from build123d import *

# Parameters (mm, degrees)
SKETCH1_R             = 5.5
SKETCH1_R_2           = 4.5
BOSS_EXTRUDE1_DEPTH   = 14
SKETCH1_R_3           = 3.5
SKETCH1_R_4           = 2.5
BOSS_EXTRUDE1_2_DEPTH = 14
SKETCH1_3_W           = 12
SKETCH1_3_H           = 11.5
BOSS_EXTRUDE2_DEPTH   = 19
FILLET1_R             = 0.2
CUT_EXTRUDE1_DEPTH    = 17
FILLET3_R             = 1
SKETCH3_R             = 1.1
SKETCH3_R_2           = 0.6
BOSS_EXTRUDE3_DEPTH   = 3.4


with BuildPart() as part:
    # Sketch1 → Boss-Extrude1 (new body)
    with BuildSketch(Plane.XY):
        Circle(SKETCH1_R)
        Circle(SKETCH1_R_2, mode=Mode.SUBTRACT)
    extrude(amount=BOSS_EXTRUDE1_DEPTH)



with BuildPart() as body_2:
    # Sketch1 → Boss-Extrude1 2 (new body)
    with BuildSketch(Plane.XY):
        Circle(SKETCH1_R_3)
        Circle(SKETCH1_R_4, mode=Mode.SUBTRACT)
    extrude(amount=BOSS_EXTRUDE1_2_DEPTH)


with BuildPart() as part_1:
    add(part.part)

    add(body_2.part)  # Boss-Extrude2 merges body 2
    # Sketch1_3 → Boss-Extrude2 (add)
    with BuildSketch(Plane.XY):
        with Locations((0, 0.25)):
            Rectangle(SKETCH1_3_W, SKETCH1_3_H)
    extrude(amount=-BOSS_EXTRUDE2_DEPTH)

    # Fillet1
    fillet1_edges = [part_1.edges().sort_by_distance(p)[0] for p in [
        (-2.5, 0, 14),
        (-3.5, 0, 14),
        (-4.5, 0, 14),
        (-5.5, 0, 14),
    ]]
    fillet(fillet1_edges, radius=FILLET1_R)

    # Sketch2 → Cut-Extrude1 (cut)
    with BuildSketch(Plane(origin=(0, 0, -19), x_dir=(-1, 0, 0), z_dir=(0, 0, -1))):
        with BuildLine():
            Line((-8.747422549, 11), (-8.747422549, 1))
            Line((-8.747422549, 1), (-6, 1))
            Line((-6, 1), (-6, 3))
            ThreePointArc((-6, 3), (-5.121320344, 5.121320344), (-3, 6))
            Line((-3, 6), (3, 6))
            ThreePointArc((3, 6), (5.121320344, 5.121320344), (6, 3))
            Line((6, 3), (6, 1))
            Line((6, 1), (7.98389041, 1))
            Line((7.98389041, 1), (7.98389041, 11))
            Line((7.98389041, 11), (-8.747422549, 11))
        make_face()
    extrude(amount=-CUT_EXTRUDE1_DEPTH, mode=Mode.SUBTRACT)

    # Fillet3
    fillet3_edges = [part_1.edges().sort_by_distance(p)[0] for p in [
        (-6, -1.25, -19),
        (0, 6, -19),
        (-5.121320344, 5.121320344, -19),
        (5.121320344, 5.121320344, -19),
        (6, -1.25, -19),
    ]]
    fillet(fillet3_edges, radius=FILLET3_R)

    # Sketch3 → Boss-Extrude3 (add)
    with BuildSketch(Plane.XZ.offset(5.5)):
        with Locations(Location((0, -13.5, 0), (0, 0, 270))):
            Circle(SKETCH3_R)
        with Locations(Location((5.08, -17.3, 0), (0, 0, 270))):
            Circle(SKETCH3_R_2)
        with Locations(Location((-5.08, -7.14, 0), (0, 0, 90))):
            Circle(SKETCH3_R_2)
        with Locations(Location((-5.08, -17.3, 0), (0, 0, 90))):
            Circle(SKETCH3_R_2)
        with Locations(Location((5.08, -7.14, 0), (0, 0, 270))):
            Circle(SKETCH3_R_2)
    extrude(amount=BOSS_EXTRUDE3_DEPTH)


solid = part_1.part
Geometry: final body of the model. Coordinates: model frame, mm. A direction names the side the tool comes from. Give positions to 0.01 mm unless a question says otherwise; leave off trailing zeros. Write each loop counter-clockwise with the first axis right and the second up, starting at its lowest first coordinate (ties: lowest second). Pieces come first, ordered by that corner, then holes. Notation, with made-up numbers: M 31.25,43 L 74.25,43 A16 cw 74.25,52 Z; hole C -2,-14.5 d8. An arc over 180 degrees is marked long. Answer in a Markdown table with one row per item. Add a question column.
(1) Section B-B on z = -7.14. Return loops of the section in (x, y).
(2) Mould query, pull axis Y, two halves, no side actions, for faces 4 (the flat face through (0, -5, 14)), 5 (the cylindrical face through (-0.59, 4.46, 6.8)), 6 (the cylindrical face through (-1.19, -5.37, 6.8)), 7 (the cylindrical face through (-0.54, -2.44, 6.8)). Classes: +Y half, -Y half, draft (parallel to the pull), parting line (faces both ways), or undercut.
(3) Reachability of faces 1 (the flat face through (-5.3, 5.4, -2)), 2 (the flat face through (0, 0, 0)), 3 (the flat face through (5.4, 5.3, -2)) from +Z, -Z, +X, -X, +Y, -Y: full face, straight path, thin tool, end or side. Return the list, or none.
(4) Section C-C on z = 4. Return loops of the section in (x, y).
(5) Ray query, line 1 (Y direction, x = 0, z = 11); line 2 (X direction, y = 2, z = 6.5); line 3 (Z direction, x = -4.5, y = -4). Return the intervals inside material, ascending.
(6) Section A-A on y = -7.5. Return loops of the section in (x, z), and give its area (3 significant figures).
(7) First-contact query: pin 1 (4 mm diameter, centred on x = -0.5, y = -1, fed in from +Z); pin 2 (2 mm diameter, centred on y = -0.5, z = 3.5, fed in from +X); pin 3 (2 mm diameter, centred on x = 0, z = 9.5, fed in from -Y); pin 4 (2.5 mm diameter, centred on x = 0, y = 1, fed in from +Z). Flat tips, straight axial feed; report the tip coordinate or a pass-through.
Result set:
| question | item | result |
|---|---|---|
| 1 | outline | M -6,-5.5 L -5.68,-5.5 L -5.68,-8.9 L -4.48,-8.9 L -4.48,-5.5 L 4.48,-5.5 L 4.48,-8.9 L 5.68,-8.9 L 5.68,-5.5 L 6,-5.5 L 6,3 A3 ccw 3,6 L -3,6 A3 ccw -6,3 Z |
| 2 | face 4 | draft |
| 2 | face 5 | undercut |
| 2 | face 6 | parting line |
| 2 | face 7 | undercut |
| 3 | face 1 | -Z, -X, +Y |
| 3 | face 2 | +Z |
| 3 | face 3 | -Z, +X, +Y |
| 4 | outline | C 0,0 d11; C 0,0 d7; hole C 0,0 d9; hole C 0,0 d5 |
| 5 | line 1 | y = -5.5 to -4.5, -3.5 to -2.5, 2.5 to 3.5, 4.5 to 5.5 |
| 5 | line 2 | x = -5.12 to -4.03, -2.87 to -1.5, 1.5 to 2.87, 4.03 to 5.12 |
| 5 | line 3 | z = -19 to 0 |
| 6 | outline | C -5.08,-17.3 d1.2; C -5.08,-7.14 d1.2; C 0,-13.5 d2.2; C 5.08,-17.3 d1.2; C 5.08,-7.14 d1.2 |
| 6 | area | 8.33 mm^2 |
| 7 | pin 1 | stops at z = 14 |
| 7 | pin 2 | stops at x = 5.5 |
| 7 | pin 3 | stops at y = -5.5 |
| 7 | pin 4 | stops at z = 0 |
